Part model, mm, in its own coordinate system. Face numbers are marked on the shaded views. A direction names the side the tool comes from. Give positions to 0.01 mm unless a question says otherwise; leave off trailing zeros. Order: outer loops, then holes, each group sorted by start corner. A loop starts at its lowest first (then second) coordinate and runs counter-clockwise, first axis right, second up.
1. Slice it at B-B on x = -4.75. List the corners of the cut face in (y, z), and give its area (3 significant figures).
2. Slice it at A-A on z = 2.75. List the corners of the cut face in (x, y), and give its area (3 significant figures).
3. Probe line 1 (X direction, y = 0.5, z = 7); line 2 (Y direction, x = -4.75, z = -6.5); line 3 (X direction, y = 2.25, z = 3.25). List the from-to ranges inside material, lowest first.
4. Which spindle directions (+Z, -Z, +X, -X, +Y, -Y) get a long thin tool onto all of the face, cutting with end or side? Do the marked faces 1, 2 and 3. Say none if no direction does.
5. Drop flat-ended pins along their axis: pin 1 Ø2 at (y, z) = (5.5, 1.5) entering from +X; pin 2 Ø1 at (x, z) = (7.5, -1) entering from +Y; pin 3 Ø3 at (x, z) = (9.23, -4.76) entering from +Y (3 decimals); pin 4 Ø1 at (x, y) = (0, 5) entering from -Z. Give the stop position or say it passes through.
6. Slice it at C-C on y = 1. List the corners of the cut face in (x, z).
7. Slice it at D-D on y = 3.5. List the corners of the cut face in (x, z), and give its area (3 significant figures).
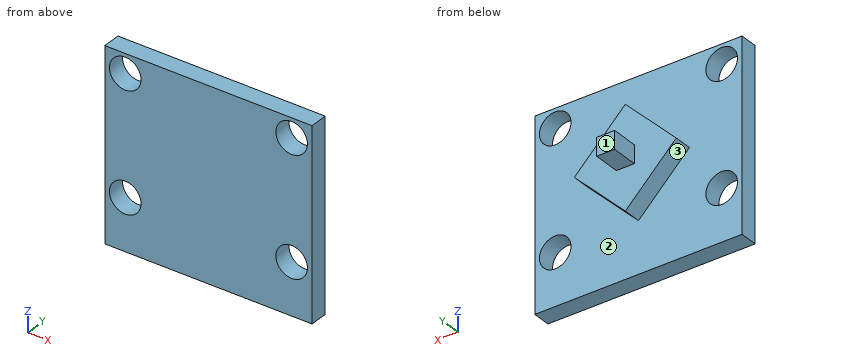
from build123d import *

# Parameters (mm, degrees)
SKETCH1_W           = 23
SKETCH1_H           = 21
BOSS_EXTRUDE1_DEPTH = 2
SKETCH2_R           = 1.75
CUT_EXTRUDE1_DEPTH  = 16.700318468
BOSS_EXTRUDE2_DEPTH = 2
SKETCH4_W           = 2
SKETCH4_H           = 2
BOSS_EXTRUDE3_DEPTH = 3


with BuildPart() as part:
    # Sketch1 → Boss-Extrude1 (new body)
    with BuildSketch(Plane(origin=(0, 0, 0), x_dir=(1, 0, 0), z_dir=(0, 1, 0))):
        Rectangle(SKETCH1_W, SKETCH1_H)
    extrude(amount=BOSS_EXTRUDE1_DEPTH)

    # Sketch2 → Cut-Extrude1 (cut, through all)
    with BuildSketch(Plane(origin=(0, 2, 0), x_dir=(1, 0, 0), z_dir=(0, 1, 0))):
        with Locations(Location((-9.233302989, -8.367680834, 0), (0, 0, 270))):
            Circle(SKETCH2_R)
        with Locations(Location((9.233302989, -8.367680834, 0), (0, 0, 270))):
            Circle(SKETCH2_R)
        with Locations(Location((9.233302989, 4.764127862, 0), (0, 0, 270))):
            Circle(SKETCH2_R)
        with Locations(Location((-9.233302989, 4.764127862, 0), (0, 0, 270))):
            Circle(SKETCH2_R)
    extrude(amount=-CUT_EXTRUDE1_DEPTH, mode=Mode.SUBTRACT)

    # Sketch3 → Boss-Extrude2 (add)
    with BuildSketch(Plane(origin=(0, 2, 0), x_dir=(1, 0, 0), z_dir=(0, 1, 0))):
        Polygon((-5.656854249, -0.843145751), (0, -6.5), (5.656854249, -0.843145751), (0, 4.813708499), align=None)
    extrude(amount=BOSS_EXTRUDE2_DEPTH)

    # Sketch4 → Boss-Extrude3 (add)
    with BuildSketch(Plane(origin=(0, 4, 0), x_dir=(1, 0, 0), z_dir=(0, 1, 0))):
        with Locations((0, -0.843145751)):
            Rectangle(SKETCH4_W, SKETCH4_H)
    extrude(amount=BOSS_EXTRUDE3_DEPTH)


solid = part.part
Data:
1. outline: (0, -10.5) - (2, -10.5) - (2, -0.06) - (4, -0.06) - (4, 1.75) - (2, 1.75) - (2, 10.5) - (0, 10.5) - close
1. area: 45.6 mm2
2. outline: (-11.5, 0) - (11.5, 0) - (11.5, 2) - (3.75, 2) - (3.75, 4) - (-3.75, 4) - (-3.75, 2) - (-11.5, 2) - close
2. area: 61.0 mm2
3. line 1: x = -11.5 to -10.33, -8.14 to 8.14, 10.33 to 11.5
3. line 2: y = 0 to 2
3. line 3: x = -3.25 to 3.25
4. face 1: +Z, -Z, +X, -X, +Y
4. face 2: +Y
4. face 3: -Z, -X, +Y
5. pin 1: stops at x = 1
5. pin 2: stops at y = 2
5. pin 3: passes through
5. pin 4: stops at z = -0.16
6. outline: (-11.5, -10.5) - (11.5, -10.5) - (11.5, 10.5) - (-11.5, 10.5) - close; hole circle Ø3.5 at (-9.23, -4.76); hole circle Ø3.5 at (-9.23, 8.37); hole circle Ø3.5 at (9.23, -4.76); hole circle Ø3.5 at (9.23, 8.37)
7. outline: (-5.66, 0.84) - (0, -4.81) - (5.66, 0.84) - (0, 6.5) - close
7. area: 64.0 mm2
